Design review of the part shown in the three views and the two pictorial views. Dimensions are in mm from the part's minimum x, y and z. A direction names the side the tool comes from. Round coordinates to 2 decimals unless told otherwise and drop trailing zeros. Loops run counter-clockwise (first coordinate to the right, second up) from the corner with the lowest first, then second, coordinate; pieces in that order, holes last.
1. Clearance check with flat-ended pins moving along their axes: pin 1 Ø2 at (y, z) = (6, 2.5) entering from -X; pin 2 Ø8 at (y, z) = (5, 15.5) entering from -X; pin 3 Ø4 at (x, y) = (4.5, 4) entering from +Z. State where each tip first meets the part, or that it passes through.
2. To check wall thickness, follow line 1 along Y through (x, z) = (15.75, 11.5); line 2 along Z through (x, y) = (3.25, 4.25); line 3 along X through (y, z) = (12.75, 7.5). State the ranges of each line that lie inside material, in increasing order.
3. Tool access review of the marked faces 1 and 2: name each direction out of +Z, -Z, +X, -X, +Y, -Y from which nothing blocks a thin tool from reaching the whole face with its end or side.
4. Consider section A-A on z = 10. State the section outline as (x, y) points.
5. Consider section D-D on z = 18.75. State the section outline as (x, y) points, then the cut area to 3 significant figures.
6. Consider section C-C on y = 6.75. State the section outline as (x, z) points.
7. Consider section B-B on x = 3.25. State the section outline as (y, z) points, then the cut area to 3 significant figures.
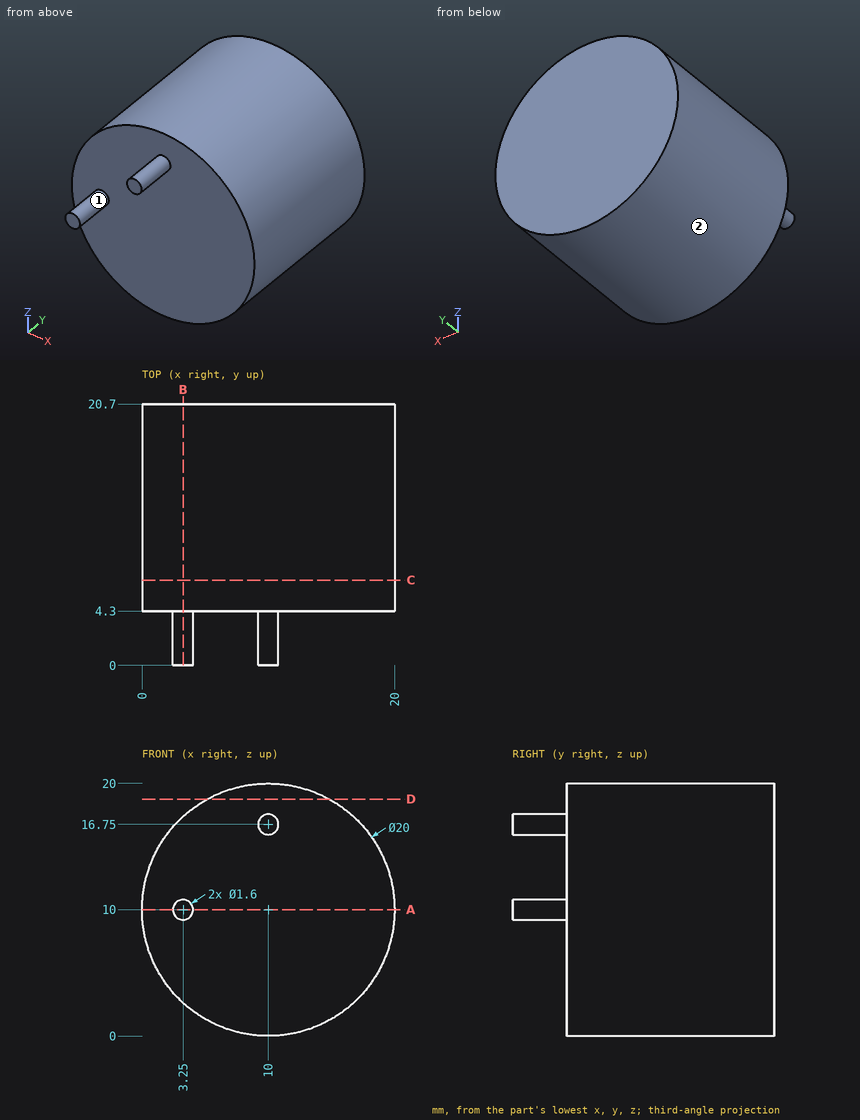
Resolved:
1. pin 1: stops at x = 2.4
1. pin 2: stops at x = 0.11
1. pin 3: stops at z = 19.36
2. line 1: y = 4.3 to 20.7
2. line 2: z = 9.2 to 10.8
2. line 3: x = 0.32 to 19.68
3. face 1: -Y
3. face 2: +Y, -Y
4. outline: (0, 4.3) - (2.45, 4.3) - (2.45, 0) - (4.05, 0) - (4.05, 4.3) - (20, 4.3) - (20, 20.7) - (0, 20.7) - close
5. outline: (5.16, 4.3) - (14.84, 4.3) - (14.84, 20.7) - (5.16, 20.7) - close
5. area: 159 mm2
6. outline: circle Ø20 at (10, 10)
7. outline: (0, 9.2) - (4.3, 9.2) - (4.3, 2.62) - (20.7, 2.62) - (20.7, 17.38) - (4.3, 17.38) - (4.3, 10.8) - (0, 10.8) - close
7. area: 249 mm2
